Geometry check sheet. Reference: the model listing, model coordinates, mm. Face numbers are marked on the shaded views. A direction names the side the tool comes from. Coordinates: 2 decimals unless noted, no trailing zeros. Loops run counter-clockwise (first coordinate to the right, second up) from the corner with the lowest first, then second, coordinate; pieces in that order, holes last. Notation, with made-up numbers: (-32.5, -27) - (-22.5, -27) arc R22 cw to (-22.5, 12) - close; hole circle Ø5 at (34.25, 30.25). An arc over 180 degrees is marked (long way). Write each question's results on one line, items separated by ' | '. Start each with the question number.
(1) Sectioned sample at A-A (y = 38.1). Enter the section's corners in (x, z), plus the area to 3 significant figures.
(2) Material ranges on probe 1 along Z at (x, y) = (72.5, 40); probe 2 along X at (y, z) = (38, -109.5); probe 3 along Z at (x, y) = (35.5, 72), recorded low to high.
(3) Access from +Z, -Z, +X, -X, +Y, -Y to the whole of each face (thin tool, end or side, straight path). Record for the marked faces 1 and 2.
(4) Go/stop test with flat-tipped pins: pin 1 Ø4 at (y, z) = (42.5, -70.5) entering from +X; pin 2 Ø4 at (x, y) = (-48, 66.5) entering from -Z; pin 3 Ø6 at (y, z) = (43, -104.5) entering from -X. Record where each tip stops, or that it passes through.
(5) Sectioned sample at C-C (z = -54.5). Enter the section's corners in (x, y), plus the area to 3 significant figures.
(6) Sectioned sample at D-D (x = 21). Enter the section's corners in (y, z), plus the area to 3 significant figures.
(7) Sectioned sample at B-B (x = 59.69). Enter the section's corners in (y, z).
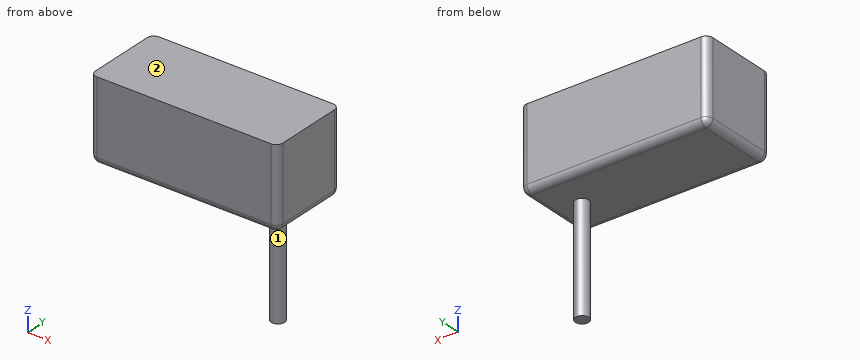
from build123d import *

# Parameters (mm, degrees)
SKETCH1_W           = 177.8
SKETCH1_H           = 76.2
BOSS_EXTRUDE1_DEPTH = 76.2
FILLET1_R           = 6.35
SKETCH2_R           = 6.35
BOSS_EXTRUDE2_DEPTH = 101.6
FILLET2_R           = 6.35


with BuildPart() as part:
    # Sketch1 → Boss-Extrude1 (new body)
    with BuildSketch(Plane(origin=(0, 0, 0), x_dir=(1, 0, 0), z_dir=(0, 1, 0))):
        Rectangle(SKETCH1_W, SKETCH1_H)
    extrude(amount=BOSS_EXTRUDE1_DEPTH)

    # Fillet1
    fillet1_edges = [part.edges().sort_by_distance(p)[0] for p in [
        (88.9, 76.2, 0),
        (-88.9, 76.2, 0),
        (88.9, 0, 0),
        (-88.9, 0, 0),
    ]]
    fillet(fillet1_edges, radius=FILLET1_R)

    # Sketch2 → Boss-Extrude2 (add)
    with BuildSketch(Plane(origin=(0, 0, -38.1), x_dir=(-1, 0, 0), z_dir=(0, 0, -1))):
        with Locations(Location((-59.69, 38.1, 0), (0, 0, 180))):
            Circle(SKETCH2_R)
    extrude(amount=BOSS_EXTRUDE2_DEPTH)

    # Fillet2
    fillet2_edges = [part.edges().sort_by_distance(p)[0] for p in [
        (-88.9, 38.1, -38.1),
        (0, 0, -38.1),
        (0, 76.2, -38.1),
        (88.9, 38.1, -38.1),
        (87.040128061, 74.340128061, -38.1),
        (-87.040128061, 74.340128061, -38.1),
        (87.040128061, 1.859871939, -38.1),
        (-87.040128061, 1.859871939, -38.1),
    ]]
    fillet(fillet2_edges, radius=FILLET2_R)


solid = part.part
Outcome:
1) outline: (-88.9, -31.75) arc R6.35 ccw to (-82.55, -38.1) - (53.34, -38.1) - (53.34, -139.7) - (66.04, -139.7) - (66.04, -38.1) - (82.55, -38.1) arc R6.35 ccw to (88.9, -31.75) - (88.9, 38.1) - (-88.9, 38.1) - close | area: 14,800 mm2
2) probe 1: z = -38.1 to 38.1 | probe 2: x = 53.34 to 66.04 | probe 3: z = -37.72 to 38.1
3) face 1: -Z | face 2: +Z, +X, -X, +Y, -Y
4) pin 1: stops at x = 65.57 | pin 2: stops at z = -38.1 | pin 3: stops at x = 53.63
5) outline: circle Ø12.7 at (59.69, 38.1) | area: 127 mm2
6) outline: (0, -31.75) arc R6.35 ccw to (6.35, -38.1) - (69.85, -38.1) arc R6.35 ccw to (76.2, -31.75) - (76.2, 38.1) - (0, 38.1) - close | area: 5,790 mm2
7) outline: (0, -31.75) arc R6.35 ccw to (6.35, -38.1) - (31.75, -38.1) - (31.75, -139.7) - (44.45, -139.7) - (44.45, -38.1) - (69.85, -38.1) arc R6.35 ccw to (76.2, -31.75) - (76.2, 38.1) - (0, 38.1) - close
